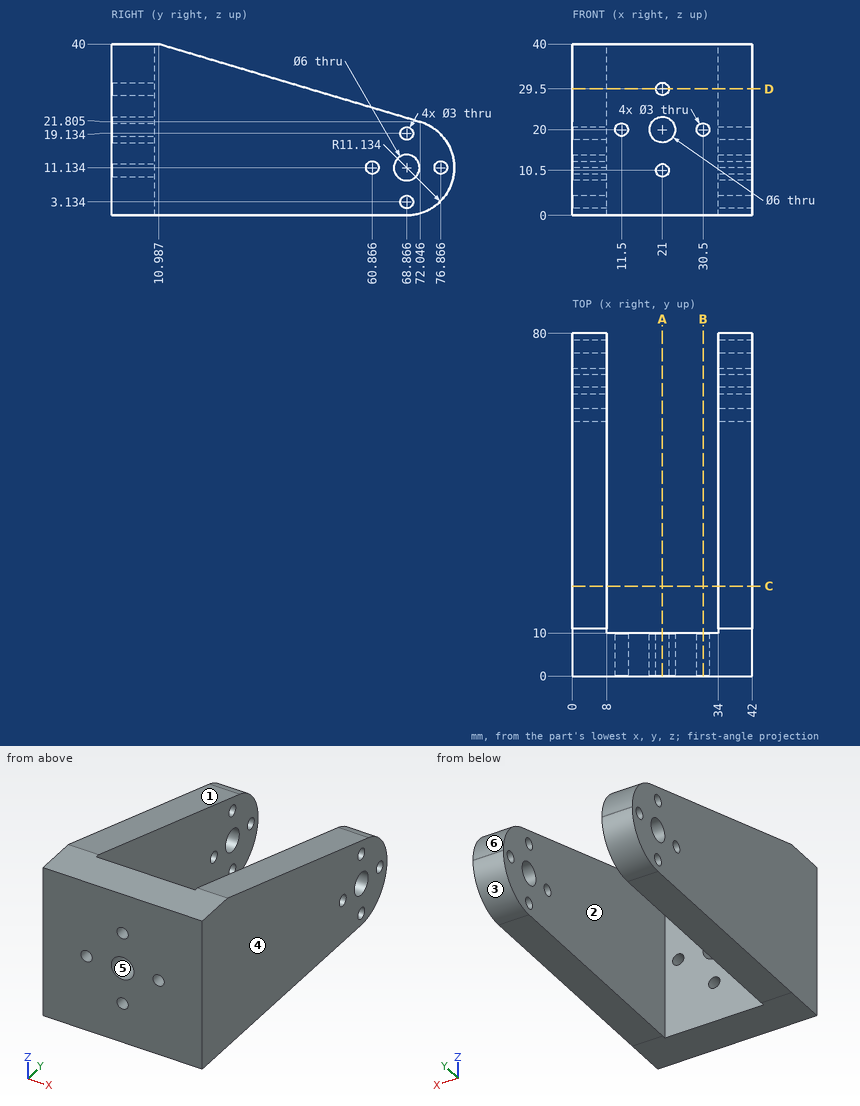
Drawing for the job (mm, zero at the part's lowest x, y, z). A direction names the side the tool comes from. Round coordinates to 2 decimals unless told otherwise and drop trailing zeros. Loops run counter-clockwise (first coordinate to the right, second up) from the corner with the lowest first, then second, coordinate; pieces in that order, holes last.
1. Band-saw the part on D-D, the plane z = 29.5. List the corners of the cut face in (x, y).
Check values:
outline: (0, 0) - (19.5, 0) - (19.5, 10) - (8, 10) - (8, 46.22) - (0, 46.22) - close; (22.5, 0) - (42, 0) - (42, 46.22) - (34, 46.22) - (34, 10) - (22.5, 10) - close
2. Drop flat-ended pins along their axis: P1, Ø8, axis at x = 23.5, z = 14.5, coming from the +Y side; P2, Ø10, axis at x = 5.5, z = 17, coming from the +Y side. Give the stop position or say it passes through.
Check values:
P1: stops at y = 10
P2: stops at y = 79.97
3. Mould opens along Z. For the marked faces 3, 4, 5 and 6 say: +Z half, -Z half, draft (parallel to the pull), parting line (faces both ways), or undercut.
Check values:
face 3: -Z half
face 4: draft
face 5: undercut
face 6: +Z half
4. Tool access for the marked faces 1 and 2: list every direction of +Z, -Z, +X, -X, +Y, -Y with a clear straight run to the whole face (end or side of a thin tool).
Check values:
face 1: +Z, +X, -X, +Y
face 2: +Z, -Z, +Y
5. Band-saw the part on C-C, the plane y = 21. List the corners of the cut face in (x, z).
Check values:
outline: (0, 0) - (8, 0) - (8, 37.02) - (0, 37.02) - close; (34, 0) - (42, 0) - (42, 37.02) - (34, 37.02) - close
6. Band-saw the part on A-A, the plane x = 21. List the corners of the cut face in (y, z), and give its area (3 significant figures).
Check values:
outline: (0, 0) - (10, 0) - (10, 9) - (0, 9) - close; (0, 12) - (10, 12) - (10, 17) - (0, 17) - close; (0, 23) - (10, 23) - (10, 28) - (0, 28) - close; (0, 31) - (10, 31) - (10, 40) - (0, 40) - close
area: 280 mm2
7. Band-saw the part on B-B, the plane x = 30.5. List the corners of the cut face in (y, z), and give its area (3 significant figures).
Check values:
outline: (0, 0) - (10, 0) - (10, 18.5) - (0, 18.5) - close; (0, 21.5) - (10, 21.5) - (10, 40) - (0, 40) - close
area: 370 mm2
8. Wall check: probe 1 along X at (y, z) = (5, 20); probe 2 along X at (y, z) = (50, 18); probe 3 along X at (y, z) = (3.75, 10.5). Give the ranges that are in metal, low to high.
Check values:
probe 1: x = 0 to 10, 13 to 18, 24 to 29, 32 to 42
probe 2: x = 0 to 8, 34 to 42
probe 3: x = 0 to 19.5, 22.5 to 42
